Work out the finished part from the listing and answer in its coordinate system (mm). A direction names the side the tool comes from. Coordinates: 2 decimals unless noted, no trailing zeros. Loops run counter-clockwise (first coordinate to the right, second up) from the corner with the lowest first, then second, coordinate; pieces in that order, holes last.
```python
from build123d import *

# Parameters (mm, degrees)
SKETCH1_R               = 1.9
SKETCH1_R_2             = 5.01
BOSS_EXTRUDE1_DEPTH     = 8
SKETCH2_R               = 1.9
BOSS_EXTRUDE2_DEPTH     = 3
SKETCH3_R               = 1.4
CUT_EXTRUDE1_DEPTH      = 22
CUT_EXTRUDE3_DEPTH      = 8
MIRROR3_COPY_1_SKETCH_R = 1.4
MIRROR3_COPY_1_DEPTH    = 22


with BuildPart() as part:
    # Sketch1 → Boss-Extrude1 (new body)
    with BuildSketch(Plane(origin=(0, 0, 0), x_dir=(1, 0, 0), z_dir=(0, 1, 0))):
        with BuildLine():
            Line((-9.451570228, 3.266162922), (-3.515864775, 20.442812793))
            ThreePointArc((-3.515864775, 20.442812793), (6.49200509, 26.385607509), (14.01, 17.5))
            Line((14.01, 17.5), (7.962554998, 0))
            Line((7.962554998, 0), (14.01, -17.5))
            ThreePointArc((14.01, -17.5), (6.49200509, -26.385607509), (-3.515864775, -20.442812793))
            Line((-3.515864775, -20.442812793), (-9.451570228, -3.266162922))
            ThreePointArc((-9.451570228, -3.266162922), (-10, 0), (-9.451570228, 3.266162922))
        make_face()
        with Locations(Location((0, 0, 0), (0, 0, 270))):
            Circle(SKETCH1_R, mode=Mode.SUBTRACT)
        with Locations(Location((5, 17.5, 0), (0, 0, 270))):
            Circle(SKETCH1_R_2, mode=Mode.SUBTRACT)
        with Locations(Location((5, -17.5, 0), (0, 0, 270))):
            Circle(SKETCH1_R_2, mode=Mode.SUBTRACT)
    extrude(amount=BOSS_EXTRUDE1_DEPTH)

    # Sketch2 → Boss-Extrude2 (add)
    with BuildSketch(Plane(origin=(0, 0, 0), x_dir=(1, 0, 0), z_dir=(0, 1, 0))):
        with BuildLine():
            Line((13.381079467, 20.80720531), (16.642446553, 25.488071975))
            ThreePointArc((16.642446553, 25.488071975), (16.031174239, 30.634605863), (10.84846826, 30.629744064))
            Line((10.84846826, 30.629744064), (6.141997733, 26.43733412))
            Line((6.141997733, 26.43733412), (13.381079467, 20.80720531))
        make_face()
        with Locations(Location((13.442555379, 27.717577856, 0), (0, 0, 270))):
            Circle(SKETCH2_R, mode=Mode.SUBTRACT)
    boss_extrude2 = extrude(amount=BOSS_EXTRUDE2_DEPTH)

    # Sketch3 → Cut-Extrude1 (cut)
    with BuildSketch(Plane(origin=(7.113123944, 0, 2.458070049), x_dir=(0.3266162922151865, 0, -0.9451570227531528), z_dir=(0.9451570227531528, 0, 0.3266162922151865))):
        with Locations((18.173329359, 4)):
            Circle(SKETCH3_R)
    cut_extrude1 = extrude(amount=-CUT_EXTRUDE1_DEPTH, mode=Mode.SUBTRACT)

    # Mirror1: Cut-Extrude1 across plane
    add(cut_extrude1.mirror(Plane.XY), mode=Mode.SUBTRACT)

    # Sketch5 → Cut-Extrude3 (cut)
    with BuildSketch(Plane(origin=(0, 0, 0), x_dir=(1, 0, 0), z_dir=(0, 1, 0))):
        Polygon((-2.052506292, 12.430669751), (-4.202841327, 6.208064486), (5.87576418, 6.208064486), align=None)
    cut_extrude3 = extrude(amount=CUT_EXTRUDE3_DEPTH, mode=Mode.SUBTRACT)

    # Mirror3: Boss-Extrude2, Cut-Extrude1, Cut-Extrude3 across plane
    add(boss_extrude2.mirror(Plane.XY))
    add(cut_extrude1.mirror(Plane.XY), mode=Mode.SUBTRACT)
    add(cut_extrude3.mirror(Plane.XY), mode=Mode.SUBTRACT)

    # Mirror3 copy 1 sketch → Mirror3 copy 1 (cut)
    with BuildSketch(Plane(origin=(7.113123944, 0, 2.458070049), x_dir=(0.3266162922151865, 0, -0.9451570227531528), z_dir=(0.9451570227531528, 0, 0.3266162922151865))):
        with Locations((18.173329359, 4)):
            Circle(MIRROR3_COPY_1_SKETCH_R)
    extrude(amount=-MIRROR3_COPY_1_DEPTH, mode=Mode.SUBTRACT)


solid = part.part
```
1. A cutting plane is placed at A-A, the plane y = 6. Give the vertices of the cut face in (x, z).
2. A cutting plane is placed at B-B, the plane x = -8.25. Give the vertices of the cut face in (y, z).
3. For faces 1 (the flat face through (12, 3, -26)), 2 (the flat face through (1, 4, -6.208)), 3 (the flat face through (-6.442, 3.944, 11.975)), 4 (the flat face through (10.944, 3.944, 8.628)), determine the directions among +Z, -Z, +X, -X, +Y, -Y from which every point of the face is accessible in a straight line to the end or side of a thin tool.
4. Each of these flat-tipped pins is pushed along its axis until it touches: P1, Ø4, axis at x = -3.5, y = 6, coming from the +Z side; P2, Ø2, axis at x = 0, y = 2.5, coming from the +Z side; P3, Ø2.5, axis at x = 3, y = 3, coming from the -Z side; P4, Ø6, axis at x = 5, z = -17.5, coming from the -Y side. Where does it stop, or does it pass through?
5. Straight lines are drawn through the part: probe 1 along Z at (x, y) = (7, 7.75); probe 2 along X at (y, z) = (3.75, 0); probe 3 along Z at (x, y) = (2.75, 1). For each, find the intervals that lie inside material, in ascending order.
6. Determine the mould class of faces 5 (the flat face through (2.2, 8, -0.4)), 6 (the cylindrical face through (11.22, 2.633, -15.029)), 7 (the flat face through (8.528, 1.479, 28.563)) for opening direction Y: released by +Y, released by -Y, zero draft, split by the parting line, or undercut.
Answers below:
1. outline: (-9.45, -3.27) - (-3.52, -20.44) arc R9.01 ccw to (14.01, -17.5) - (7.96, 0) - (14.01, 17.5) arc R9.01 ccw to (-3.52, 20.44) - (-9.45, 3.27) arc R10 ccw to start; hole (-4.2, -6.21) - (-2.05, -12.43) - (5.88, -6.21) - close; hole (-4.2, 6.21) - (5.88, 6.21) - (-2.05, 12.43) - close; hole circle Ø3.8 at (0, 0); hole circle Ø10.02 at (5, -17.5); hole circle Ø10.02 at (5, 17.5)
2. outline: (0, -6.74) - (8, -6.74) - (8, 6.74) - (0, 6.74) - close
3. face 1: -Z, +X, +Y
3. face 2: +Y, -Y
3. face 3: +Z, -X, +Y, -Y
3. face 4: +X, +Y, -Y
4. P1: stops at z = 23.74
4. P2: stops at z = 25.57
4. P3: stops at z = -26.48
4. P4: passes through
5. probe 1: z = -26.29 to -22.09, -12.91 to 12.91, 22.09 to 26.29
5. probe 2: x = -10 to -1.9, 1.9 to 7.96
5. probe 3: z = -26.22 to -21.98, -13.02 to -8.66, -6.21 to 6.21, 8.66 to 13.02, 21.98 to 26.22
6. face 5: released by +Y
6. face 6: undercut
6. face 7: zero draft
